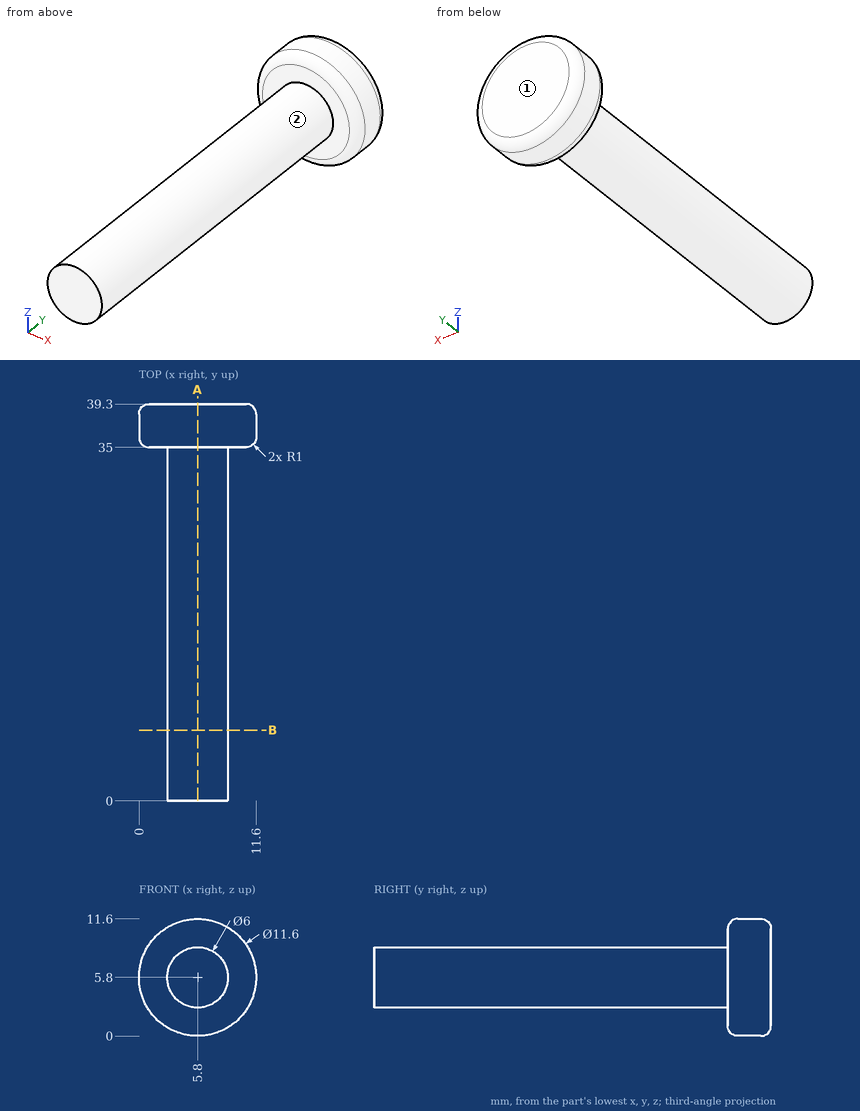
The drawing under review shows one solid part. Ordinate dimensions are in mm from its lowest x, y, z. A direction names the side the tool comes from. Round coordinates to 2 decimals unless told otherwise and drop trailing zeros. Loops run counter-clockwise (first coordinate to the right, second up) from the corner with the lowest first, then second, coordinate; pieces in that order, holes last. Notation, with made-up numbers: (-0.75, 6.5) - (5.25, 6.5) arc R19 ccw to (5.25, 16.5) - close; hole circle Ø9 at (39, 2). An arc over 180 degrees is marked (long way). Put each result on its own line as item: value. Start each with the question number.
1. Consider section A-A on x = 5.8. State the section outline as (y, z) points, plus the area to 3 significant figures.
2. Insertion check: P1, Ø3, axis at y = 6.5, z = 5.5, coming from the -X side; P2, Ø2, axis at x = 8.5, z = 9.5, coming from the -Y side. Each pin has a flat end and moves straight along its axis. Give the tip position at first contact, or say it passes through.
3. For probe 1 along Z at (x, y) = (6, 30.5); probe 2 along Y at (x, z) = (1.5, 4), list the stretches that pass through material, from the lowest coordinate up. Write a range as [from, to].
4. For the marked faces 1 and 2, list the 3-axis set-ups (+Z, -Z, +X, -X, +Y, -Y) from which the entire face can be reached by the end or side of a thin tool; tool diameter is ignored.
5. Consider section B-B on y = 7. State the section outline as (x, z) points, plus the area to 3 significant figures.
Result sheet:
1. outline: (0, 2.8) - (35, 2.8) - (35, 1) arc R1 ccw to (36, 0) - (38.3, 0) arc R1 ccw to (39.3, 1) - (39.3, 10.6) arc R1 ccw to (38.3, 11.6) - (36, 11.6) arc R1 ccw to (35, 10.6) - (35, 8.8) - (0, 8.8) - close
1. area: 259 mm^2
2. P1: x = 2.8
2. P2: y = 35
3. probe 1: [2.81, 8.79]
3. probe 2: [35, 39.3]
4. face 1: +Z, -Z, +X, -X, +Y
4. face 2: -Y
5. outline: circle Ø6 at (5.8, 5.8)
5. area: 28.3 mm^2
